```python
from build123d import *

# Parameters (mm, degrees)
BOSS_EXTRUDE1_DEPTH = 7
SKETCH2_W           = 7
SKETCH2_H           = 46
BOSS_EXTRUDE2_DEPTH = 28
SKETCH4_R           = 6.125
CUT_EXTRUDE1_DEPTH  = 7
SKETCH5_R           = 1.75
CUT_EXTRUDE3_DEPTH  = 7
SKETCH6_W           = 10
SKETCH6_H           = 28
CUT_EXTRUDE4_DEPTH  = 10
CUT_EXTRUDE5_DEPTH  = 10
SKETCH8_R           = 2
CUT_EXTRUDE6_DEPTH  = 10


with BuildPart() as part:
    # Sketch1 → Boss-Extrude1 (new body)
    with BuildSketch(Plane(origin=(0, 0, 0), x_dir=(1, 0, 0), z_dir=(0, 1, 0))):
        with BuildLine():
            Line((25.4, 23), (25.4, -23))
            Line((25.4, -23), (0, -23))
            ThreePointArc((0, -23), (-23, 0), (0, 23))
            Line((0, 23), (25.4, 23))
        make_face()
    extrude(amount=-BOSS_EXTRUDE1_DEPTH)

    # Sketch2 → Boss-Extrude2 (add)
    with BuildSketch(Plane.XZ.offset(7)):
        with Locations((21.9, 0)):
            Rectangle(SKETCH2_W, SKETCH2_H)
    extrude(amount=BOSS_EXTRUDE2_DEPTH)

    # Sketch4 → Cut-Extrude1 (cut)
    with BuildSketch(Plane(origin=(0, 0, 0), x_dir=(1, 0, 0), z_dir=(0, 1, 0))):
        Circle(SKETCH4_R)
    extrude(amount=-CUT_EXTRUDE1_DEPTH, mode=Mode.SUBTRACT)

    # Sketch5 → Cut-Extrude3 (cut)
    with BuildSketch(Plane(origin=(0, 0, 0), x_dir=(1, 0, 0), z_dir=(0, 1, 0))):
        with Locations((-6.731, 15.621)):
            Circle(SKETCH5_R)
        with Locations((-6.731, -15.621)):
            Circle(SKETCH5_R)
    extrude(amount=-CUT_EXTRUDE3_DEPTH, mode=Mode.SUBTRACT)

    # Sketch6 → Cut-Extrude4 (cut)
    with BuildSketch(Plane.ZY.offset(-18.4)):
        with Locations((18, -21)):
            Rectangle(SKETCH6_W, SKETCH6_H)
        with Locations((-18, -21)):
            Rectangle(SKETCH6_W, SKETCH6_H)
    extrude(amount=-CUT_EXTRUDE4_DEPTH, mode=Mode.SUBTRACT)

    # Sketch7 → Cut-Extrude5 (cut)
    with BuildSketch(Plane.XZ.offset(7)):
        Polygon((0, -23), (18.4, -13), (25.4, -13), (25.4, -23), align=None)
        Polygon((0, 23), (18.4, 13), (25.4, 13), (25.4, 23), align=None)
    extrude(amount=-CUT_EXTRUDE5_DEPTH, mode=Mode.SUBTRACT)

    # Sketch8 → Cut-Extrude6 (cut)
    with BuildSketch(Plane.ZY.offset(-18.4)):
        with Locations((-8, -14)):
            Circle(SKETCH8_R)
        with Locations((8, -14)):
            Circle(SKETCH8_R)
        with Locations((-8, -28.225)):
            Circle(SKETCH8_R)
        with Locations((8, -28.225)):
            Circle(SKETCH8_R)
    extrude(amount=-CUT_EXTRUDE6_DEPTH, mode=Mode.SUBTRACT)


solid = part.part
```
Geometry check sheet. Reference: the model listing, model coordinates, mm. A direction names the side the tool comes from. Give positions to 0.01 mm unless a question says otherwise; leave off trailing zeros. Order: outer loops, then holes, each group sorted by start corner. A loop starts at its lowest first (then second) coordinate and runs counter-clockwise, first axis right, second up.
1. Section check C-C, the plane z = -2.5. Enter the section's corners in (x, y), and give its area (3 significant figures).
2. Section check B-B, the plane x = 1.5. Enter the section's corners in (y, z), and give its area (3 significant figures).
3. Access from +Z, -Z, +X, -X, +Y, -Y to the whole of each face (thin tool, end or side, straight path). Record for faces 5 (the face through (25.4, -17, 0)), 6 (the face through (22, -18, -13)), 7 (the face through (-7, -7, 0)).
4. Section check A-A, the plane y = -14. Enter the section's corners in (x, z), and give its area (3 significant figures).
5. Gauge pin test, flat ends, axial feed: pin 1 Ø6 at (y, z) = (-12.5, -8) entering from -X; pin 2 Ø5.5 at (x, z) = (-6.731, -15.621) entering from +Y; pin 3 Ø12 at (x, y) = (-16.5, -7) entering from -Z; pin 4 Ø7.5 at (x, y) = (21.5, -26) entering from -Z. Record the tip position at first contact, or that the pin passes through.
6. Thickness scan on L1, parallel to Y at x = 23, z = -8 (3 decimals); L2, parallel to Z at x = 0, y = -3 (3 decimals); L3, parallel to Y at x = -11, z = 4.5. Record the ranges inside material, lowest first.
7. Section check D-D, the plane x = 20. Enter the section's corners in (y, z) (3 decimals).
8. Release check for a two-part mould opening along Y. For faces 1 (the face through (21.85, -30.18, 7.57)), 2 (the face through (21.851, -12.648, -9.474)), 3 (the face through (22, -18, 13)), 4 (the face through (7, 0, 0)) record: pulls with the +Y half, pulls with the -Y half, needs draft (parallel to the pull), parting line crosses it, or undercut.
Values follow:
1. outline: (-22.86, -7) - (-5.59, -7) - (-5.59, 0) - (-22.86, 0) - close; (5.59, -7) - (18.4, -7) - (18.4, -35) - (25.4, -35) - (25.4, 0) - (5.59, 0) - close
1. area: 456 mm2
2. outline: (-7, -22.18) - (0, -22.18) - (0, -5.94) - (-7, -5.94) - close; (-7, 5.94) - (0, 5.94) - (0, 22.18) - (-7, 22.18) - close
2. area: 227 mm2
3. face 5: +Z, -Z, +X, +Y, -Y
3. face 6: -Z, +X, +Y, -Y
3. face 7: +Z, -Z, -X, -Y
4. outline: (18.4, -13) - (25.4, -13) - (25.4, -10) - (18.4, -10) - close; (18.4, -6) - (25.4, -6) - (25.4, 6) - (18.4, 6) - close; (18.4, 10) - (25.4, 10) - (25.4, 13) - (18.4, 13) - close
4. area: 126 mm2
5. pin 1: stops at x = 18.4
5. pin 2: stops at y = 0
5. pin 3: stops at z = -20.46
5. pin 4: stops at z = -13
6. L1: y = -35 to -30.225, -26.225 to -16, -12 to 0
6. L2: z = -23 to -6.125, 6.125 to 23
6. L3: y = -7 to 0
7. outline: (-35, -13) - (0, -13) - (0, 13) - (-35, 13) - close; hole circle Ø4 at (-28.225, -8); hole circle Ø4 at (-28.225, 8); hole circle Ø4 at (-14, -8); hole circle Ø4 at (-14, 8)
8. face 1: undercut
8. face 2: undercut
8. face 3: needs draft
8. face 4: pulls with the +Y half
